Check sheet for the modelled part. Datum: model origin and axes. Units: mm. A direction names the side the tool comes from. Round coordinates to 2 decimals unless told otherwise and drop trailing zeros. Write each loop counter-clockwise with the first axis right and the second up, starting at its lowest first coordinate (ties: lowest second). Pieces come first, ordered by that corner, then holes. Notation, with made-up numbers: (-19, 83.25) -> (26, 83.25) arc R21 cw to (26, 96.25) -> close; hole circle Ø6 at (-11.5, 54.25). An arc over 180 degrees is marked (long way). One line per item, written item: value.
Autodesk Inventor part; units mm, degrees
ref_plane "YZ Plane" through (0, 0, 0) normal (1, 0, 0) x (0, 1, 0)
ref_plane "XZ Plane" through (0, 0, 0) normal (0, 1, 0) x (-1, 0, 0)
ref_plane "XY Plane" through (0, 0, 0) normal (0, 0, 1) x (1, 0, 0)
sketch "Sketch1" plane through (0, 0, 0) normal (1, 0, 0) x (0, 1, 0)
  arc A0 (0, 6.35) -> (0, -6.35) centre (0, 0) ccw
  arc A1 (0, 12.7) -> (0, -12.7) centre (0, 0) ccw
  line L0 (0, 12.7) -> (50.8, 12.7)
  line L1 (0, -12.7) -> (50.8, -12.7)
  line L2 (0, 6.35) -> (50.8, 6.35)
  line L3 (0, -6.35) -> (50.8, -6.35)
  line L4 (50.8, -6.35) -> (50.8, -12.7)
  line L5 (50.8, 12.7) -> (50.8, 6.35)
  dimension "d0" = 12.7
  dimension "d1" = 25.4
  dimension "d2" = 50.8
extrude "Extrusion1" add sketch "Sketch1" along normal mid plane 12.7
properties part number "U_bolt"
Item 1: Sectioned sample at A-A (y = -2). Enter the section's corners in (x, z), then the cut area to 3 significant figures.
Result set:
outline: (-6.35, -12.54) -> (6.35, -12.54) -> (6.35, -6.03) -> (-6.35, -6.03) -> close; (-6.35, 6.03) -> (6.35, 6.03) -> (6.35, 12.54) -> (-6.35, 12.54) -> close
area: 165 mm^2
Item 2: Tool access check on faces 4 (the flat face through (0, 25, 6.35)), 5 (the flat face through (0, 25, -12.7)). Record the directions out of +Z, -Z, +X, -X, +Y, -Y that give a thin tool (end or side, any length) a straight path to the whole face; none if there is none.
Result set:
face 4: +X, -X, +Y
face 5: -Z, +X, -X, +Y, -Y
Item 3: Depth check by flat-ended pin: pin 1 (1 mm diameter, centred on y = 3.5, z = -4.5, fed in from -X); pin 2 (3 mm diameter, centred on x = -1, z = 8.5, fed in from -Y); pin 3 (5 mm diameter, centred on x = -1.5, z = 8.5, fed in from -Y). Enter the tip coordinate at first touch or a pass-through.
Result set:
pin 1: through
pin 2: y = -10.6
pin 3: y = -11.19
Item 4: Sectioned sample at D-D (y = 39). Enter the section's corners in (x, z), then the cut area to 3 significant figures.
Result set:
outline: (-6.35, -12.7) -> (6.35, -12.7) -> (6.35, -6.35) -> (-6.35, -6.35) -> close; (-6.35, 6.35) -> (6.35, 6.35) -> (6.35, 12.7) -> (-6.35, 12.7) -> close
area: 161 mm^2
Item 5: Sectioned sample at B-B (x = -2.5). Enter the section's corners in (y, z).
Result set:
outline: (0, -12.7) -> (50.8, -12.7) -> (50.8, -6.35) -> (0, -6.35) arc R6.35 cw to (0, 6.35) -> (50.8, 6.35) -> (50.8, 12.7) -> (0, 12.7) arc R12.7 ccw to start
Item 6: Material ranges on line 1 along Z through (x, y) = (1, 7); line 2 along Z through (x, y) = (-2.5, -5); line 3 along Y through (x, z) = (1.5, -1.5), recorded low to high.
Result set:
line 1: -12.7 to -6.35, 6.35 to 12.7
line 2: -11.67 to -3.91, 3.91 to 11.67
line 3: -12.61 to -6.17
Item 7: Sectioned sample at C-C (z = 0). Enter the section's corners in (x, y).
Result set:
outline: (-6.35, -12.7) -> (6.35, -12.7) -> (6.35, -6.35) -> (-6.35, -6.35) -> close
Item 8: Release check for a two-part mould opening along Z. For faces 1 (the flat face through (-6.35, 19, -8)), 2 (the cylindrical face through (-0.089, -12.697, -0.279)), 3 (the cylindrical face through (-0.09, -6.35, -0.14)) record: pulls with the +Z half, pulls with the -Z half, needs draft (parallel to the pull), parting line crosses it, or undercut.
Result set:
face 1: needs draft
face 2: parting line crosses it
face 3: undercut
